```python
from build123d import *

# Parameters (mm, degrees)
F0_W     = 127
F0_H     = 127
F1_DEPTH = 6.35
F2_W     = 19.05
F2_H     = 50.8
F3_DEPTH = 50.8
F4_R     = 9.525
F5_DEPTH = 73.026
F6_W     = 12.7
F6_H     = 38.1
F7_DEPTH = 25.4
F8_R     = 19.05


with BuildPart() as f1:
    # F0 (on Front) → F1 (new body)
    with BuildSketch(Plane.XZ):
        Rectangle(F0_W, F0_H)
    extrude(amount=F1_DEPTH)

    # F2 (on face) → F3 (join)
    with BuildSketch(Plane.XZ.offset(6.35)):
        Rectangle(F2_W, F2_H)
    extrude(amount=F3_DEPTH)

    # F4 (on face) → F5 (cut, through all)
    with BuildSketch(Plane(origin=(-9.525, 0, 0), x_dir=(0, -1, 0), z_dir=(-1, 0, 0))):
        with Locations((41.91, 0)):
            Circle(F4_R)
    extrude(amount=-F5_DEPTH, mode=Mode.SUBTRACT)

    # F6 (on face) → F7 (join)
    with BuildSketch(Plane(origin=(0, 0, 0), x_dir=(-1, 0, 0), z_dir=(0, 1, 0))):
        Rectangle(F6_W, F6_H)
    extrude(amount=F7_DEPTH)

    # F8
    f8_edges = [f1.edges().sort_by_distance(p)[0] for p in [
        (0, -57.15, 25.4),
        (0, -57.15, -25.4),
    ]]
    fillet(f8_edges, radius=F8_R)


solid = f1.part
```
Part model, mm, in its own coordinate system. A direction names the side the tool comes from. Round coordinates to 2 decimals unless told otherwise and drop trailing zeros. Write each loop counter-clockwise with the first axis right and the second up, starting at its lowest first coordinate (ties: lowest second). Pieces come first, ordered by that corner, then holes.
Item 1: Which spindle directions (+Z, -Z, +X, -X, +Y, -Y) get a long thin tool onto all of the face, cutting with end or side? Do faces 1 (the flat face through (-9.525, -31, 0)), 2 (the flat face through (0, -22, -25.4)), 3 (the flat face through (0, 13, -19.05)). Say none if no direction does.
Results:
face 1: +Z, -Z, -X, -Y
face 2: -Z, +X, -X, -Y
face 3: -Z, +X, -X, +Y
Item 2: Probe L1, parallel to X at y = -11.5, z = -18 (3 decimals); L2, parallel to Y at x = -54.5, z = 21.5; L3, parallel to Z at x = 2, y = -41. List the from-to ranges inside material, lowest first.
Results:
L1: x = -9.525 to 9.525
L2: y = -6.35 to 0
L3: z = -25.18 to -9.48, 9.48 to 25.18
Item 3: Cut at A-A, the plane z = 0. Give the cut face in (x, y) (3 decimals).
Results:
outline: (-63.5, -6.35) - (-9.525, -6.35) - (-9.525, -32.385) - (9.525, -32.385) - (9.525, -6.35) - (63.5, -6.35) - (63.5, 0) - (6.35, 0) - (6.35, 25.4) - (-6.35, 25.4) - (-6.35, 0) - (-63.5, 0) - close; (-9.525, -57.15) - (9.525, -57.15) - (9.525, -51.435) - (-9.525, -51.435) - close
Item 4: Cut at C-C, the plane x = 15. Give the cut face in (y, z).
Results:
outline: (-6.35, -63.5) - (0, -63.5) - (0, 63.5) - (-6.35, 63.5) - close
Item 5: Drop flat-ended pins along their axis: pin 1 Ø14 at (x, y) = (-2.5, 11) entering from +Z; pin 2 Ø1.5 at (x, y) = (-4.5, -14.5) entering from +Z; pin 3 Ø25 at (y, z) = (-41.91, 0) entering from -X (3 decimals). Give the stop position or say it passes through.
Results:
pin 1: stops at z = 19.05
pin 2: stops at z = 25.4
pin 3: stops at x = -9.525
Item 6: Cut at B-B, the plane y = -41.91. Give the cut face in (x, z) (3 decimals), plus the area to 3 significant figures.
Results:
outline: (-9.525, -25.015) - (9.525, -25.015) - (9.525, -9.525) - (-9.525, -9.525) - close; (-9.525, 9.525) - (9.525, 9.525) - (9.525, 25.015) - (-9.525, 25.015) - close
area: 590 mm2
Item 7: Cut at D-D, the plane z = -30. Give the cut face in (x, y), plus the area to 3 significant figures.
Results:
outline: (-63.5, -6.35) - (63.5, -6.35) - (63.5, 0) - (-63.5, 0) - close
area: 806 mm2
